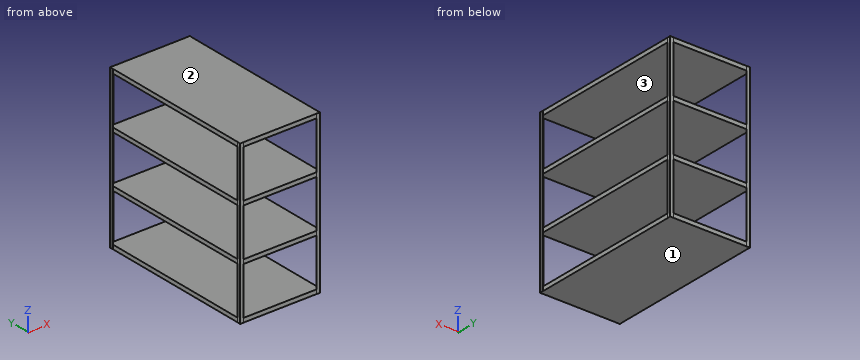
from build123d import *

# Parameters (mm, degrees)
F0_W          = 914.4
F0_H          = 1828.8
F1_DEPTH      = 47.625
F3_DEPTH      = 1781.175
F3_DEPTH_BACK = 47.625
F5_W          = 914.4
F5_H          = 1828.8
F6_DEPTH      = 47.625
F8_W          = 914.4
F8_H          = 1828.8
F9_DEPTH      = 47.625
F11_W         = 914.4
F11_H         = 1828.8
F12_DEPTH     = 47.7012


with BuildPart() as f1:
    # F0 (on Top) → F1 (new body)
    with BuildSketch(Plane.XY):
        Rectangle(F0_W, F0_H)
    extrude(amount=F1_DEPTH)

    # F2 (on face) → F3 (join, two sides)
    with BuildSketch(Plane.XY.offset(47.625)) as f3_sk:
        Polygon((458.47, -915.67), (458.47, -877.57), (457.2, -877.57), (457.2, -914.4), (420.37, -914.4), (420.37, -915.67), align=None)
        Polygon((-458.47, -915.67), (-420.37, -915.67), (-420.37, -914.4), (-457.2, -914.4), (-457.2, -877.57), (-458.47, -877.57), align=None)
        Polygon((-458.47, 915.67), (-458.47, 877.57), (-457.2, 877.57), (-457.2, 914.4), (-420.37, 914.4), (-420.37, 915.67), align=None)
        Polygon((458.47, 915.67), (420.37, 915.67), (420.37, 914.4), (457.2, 914.4), (457.2, 877.57), (458.47, 877.57), align=None)
    extrude(amount=F3_DEPTH)
    extrude(f3_sk.sketch, amount=-F3_DEPTH_BACK)

    # F5 (on offset) → F6 (join)
    with BuildSketch(Plane.XY.offset(593.725)):
        Rectangle(F5_W, F5_H)
    extrude(amount=F6_DEPTH)

    # F8 (on offset) → F9 (join)
    with BuildSketch(Plane.XY.offset(1187.45)):
        Rectangle(F8_W, F8_H)
    extrude(amount=F9_DEPTH)

    # F11 (on offset) → F12 (join)
    with BuildSketch(Plane.XY.offset(1781.175)):
        Rectangle(F11_W, F11_H)
    extrude(amount=F12_DEPTH)


solid = f1.part
Here's how the part is built. I have some questions about the finished solid (model axes, mm). Face numbers are marked on the shaded views. Round coordinates to 2 decimals unless told otherwise and drop trailing zeros. Loops run counter-clockwise (first coordinate to the right, second up) from the corner with the lowest first, then second, coordinate; pieces in that order, holes last. Notation, with made-up numbers: M 80.25,17 L 99.25,17 A22 cw 99.25,32 Z; hole C 51,-34.75 d6. An arc over 180 degrees is marked long. Write each question's results on one line, items separated by ' | '. Start each with the question number.
(1) I want a section at C-C (y = 531). Please give me the cut outline in (x, z) (3 decimals), then the cut area to 3 significant figures.
(2) I want a section at A-A (z = 207). Please give me the cut outline in (x, y), then the cut area to 3 significant figures.
(3) If I drill on probe 1 along Z at (x, y) = (-11, -739) (3 decimals); probe 2 along X at (y, z) = (114, 640); probe 3 along Y at (x, z) = (62, 631), over which ranges is the centre line in solid material (lowest first)? Write a range as from..to.
(4) I want a section at B-B (x = -307). Please give me the cut outline in (y, z) (3 decimals), then the cut area to 3 significant figures.
(5) Will these pins go through, and if not, where does the flat tip stop? P1, Ø5, axis at x = -147, y = -625.5, coming from the -Z side; P2, Ø14.5, axis at x = -13.5, z = 1222, coming from the +Y side.
(6) Thinking about a two-plate mould opening in Z: for the marked faces 1, 2 and 3, which applies, pulls with the +Z half, pulls with the -Z half, needs draft (parallel to the pull), parting line crosses it, or undercut?
Solved:
1) outline: M -457.2,0 L 457.2,0 L 457.2,47.625 L -457.2,47.625 Z; M -457.2,593.725 L 457.2,593.725 L 457.2,641.35 L -457.2,641.35 Z; M -457.2,1187.45 L 457.2,1187.45 L 457.2,1235.075 L -457.2,1235.075 Z; M -457.2,1781.175 L 457.2,1781.175 L 457.2,1828.876 L -457.2,1828.876 Z | area: 174,000 mm²
2) outline: M -458.47,-915.67 L -420.37,-915.67 L -420.37,-914.4 L -457.2,-914.4 L -457.2,-877.57 L -458.47,-877.57 Z; M -458.47,877.57 L -457.2,877.57 L -457.2,914.4 L -420.37,914.4 L -420.37,915.67 L -458.47,915.67 Z; M 420.37,-915.67 L 458.47,-915.67 L 458.47,-877.57 L 457.2,-877.57 L 457.2,-914.4 L 420.37,-914.4 Z; M 420.37,914.4 L 457.2,914.4 L 457.2,877.57 L 458.47,877.57 L 458.47,915.67 L 420.37,915.67 Z | area: 381 mm²
3) probe 1: z = 0..47.625, 593.725..641.35, 1187.45..1235.075, 1781.175..1828.876 | probe 2: x = -457.2..457.2 | probe 3: y = -914.4..914.4
4) outline: M -914.4,0 L 914.4,0 L 914.4,47.625 L -914.4,47.625 Z; M -914.4,593.725 L 914.4,593.725 L 914.4,641.35 L -914.4,641.35 Z; M -914.4,1187.45 L 914.4,1187.45 L 914.4,1235.075 L -914.4,1235.075 Z; M -914.4,1781.175 L 914.4,1781.175 L 914.4,1828.876 L -914.4,1828.876 Z | area: 349,000 mm²
5) P1: stops at z = 0 | P2: stops at y = 914.4
6) face 1: pulls with the -Z half | face 2: pulls with the +Z half | face 3: undercut
